from build123d import *

# Parameters (mm, degrees)
SKETCH1_R           = 5.5245
SKETCH1_R_2         = 1.7526
SKETCH1_W           = 12.7
SKETCH1_H           = 5.842
BOSS_EXTRUDE1_DEPTH = 5.842
FILLET1_R           = 1.5875
FILLET2_R           = 1.5875
FILLET3_R           = 3.175
CUT_EXTRUDE3_DEPTH  = 95.62556025


with BuildPart() as part:
    # Sketch1 → Boss-Extrude1 (new body)
    with BuildSketch(Plane(origin=(0, 0, 0), x_dir=(1, 0, 0), z_dir=(0, 1, 0))):
        with BuildLine():
            Line((-25.4, 57.15), (-12.411023526, -2.693788234))
            ThreePointArc((-12.411023526, -2.693788234), (-9.884908198, -7.97361837), (-5.259246403, -11.559858445))
            Line((-5.259246403, -11.559858445), (42.490805524, -33.284111388))
            Line((42.490805524, -33.284111388), (54.997863988, -35.489443244))
            Line((54.997863988, -35.489443244), (63.819191413, 14.538790609))
            Line((63.819191413, 14.538790609), (51.31213295, 16.744122465))
            Line((51.31213295, 16.744122465), (17.03122895, 18.5927693))
            Line((17.03122895, 18.5927693), (25.4, 57.15))
            Line((25.4, 57.15), (25.4, 69.85))
            Line((25.4, 69.85), (-25.4, 69.85))
            Line((-25.4, 69.85), (-25.4, 57.15))
        make_face()
        with Locations(Location((0, 0, 0), (0, 0, 270))):
            Circle(SKETCH1_R, mode=Mode.SUBTRACT)
        with Locations(Location((0, 63.5, 0), (0, 0, 270))):
            Circle(SKETCH1_R_2, mode=Mode.SUBTRACT)
        with Locations(Location((53.154998469, -9.37266039, 0), (0, 0, 270))):
            Circle(SKETCH1_R_2, mode=Mode.SUBTRACT)
        with Locations((-12.7, 63.5)):
            Rectangle(SKETCH1_W, SKETCH1_H, mode=Mode.SUBTRACT)
        with Locations((12.7, 63.5)):
            Rectangle(SKETCH1_W, SKETCH1_H, mode=Mode.SUBTRACT)
        Polygon((53.603383206, 9.991624401), (51.364030551, -2.708375599), (57.117277444, -3.722828253), (59.356630099, 8.977171747), align=None, mode=Mode.SUBTRACT)
        Polygon((52.706613732, -28.73694518), (54.945966387, -16.03694518), (49.192719493, -15.022492526), (46.953366838, -27.722492526), align=None, mode=Mode.SUBTRACT)
        with BuildLine():
            Line((-4.04068235, 18.616535288), (-11.026040035, 50.8))
            Line((-11.026040035, 50.8), (11.026040035, 50.8))
            Line((11.026040035, 50.8), (4.04068235, 18.616535288))
            ThreePointArc((4.04068235, 18.616535288), (0, 19.05), (-4.04068235, 18.616535288))
        make_face(mode=Mode.SUBTRACT)
        with BuildLine():
            Line((17.339787668, -7.888869605), (38.799209797, -17.651998555))
            Line((38.799209797, -17.651998555), (42.496670214, 3.317341488))
            Line((42.496670214, 3.317341488), (18.99222283, 1.48255589))
            ThreePointArc((18.99222283, 1.48255589), (18.760587695, -3.307997785), (17.339787668, -7.888869605))
        make_face(mode=Mode.SUBTRACT)
    extrude(amount=BOSS_EXTRUDE1_DEPTH)

    # Fillet1
    fillet1_edges = [part.edges().sort_by_distance(p)[0] for p in [
        (18.99222283, 2.921, -1.48255589),
        (17.339787668, 2.921, 7.888869605),
        (38.799209797, 2.921, 17.651998555),
        (42.496670214, 2.921, -3.317341488),
        (-4.04068235, 2.921, -18.616535288),
        (4.04068235, 2.921, -18.616535288),
        (11.026040035, 2.921, -50.8),
        (-11.026040035, 2.921, -50.8),
    ]]
    fillet(fillet1_edges, radius=FILLET1_R)

    # Fillet2
    fillet2_edges = [part.edges().sort_by_distance(p)[0] for p in [
        (-25.4, 2.921, -69.85),
        (25.4, 2.921, -69.85),
        (63.819191413, 2.921, -14.538790609),
        (54.997863988, 2.921, 35.489443244),
    ]]
    fillet(fillet2_edges, radius=FILLET2_R)

    # Fillet3
    fillet3_edges = [part.edges().sort_by_distance(p)[0] for p in [
        (25.4, 2.921, -57.15),
        (17.03122895, 2.921, -18.5927693),
        (51.31213295, 2.921, -16.744122465),
        (42.490805524, 2.921, 33.284111388),
        (-25.4, 2.921, -57.15),
    ]]
    fillet(fillet3_edges, radius=FILLET3_R)

    # Sketch2 → Cut-Extrude3 (cut, through all)
    with BuildSketch(Plane(origin=(0, 5.842, 0), x_dir=(1, 0, 0), z_dir=(0, 1, 0))):
        with BuildLine():
            Line((1.5875, 54.791775853), (-1.5875, 54.791775853))
            ThreePointArc((-1.5875, 54.791775853), (-3.96875, 57.173025853), (-1.5875, 59.554275853))
            Line((-1.5875, 59.554275853), (1.5875, 59.554275853))
            ThreePointArc((1.5875, 59.554275853), (3.96875, 57.173025853), (1.5875, 54.791775853))
        make_face()
    extrude(amount=-CUT_EXTRUDE3_DEPTH, mode=Mode.SUBTRACT)


solid = part.part
Input: part model. Units: mm. Frame: model coordinates. A direction names the side the tool comes from. Give positions to 0.01 mm unless a question says otherwise; leave off trailing zeros. Write each loop counter-clockwise with the first axis right and the second up, starting at its lowest first coordinate (ties: lowest second). Pieces come first, ordered by that corner, then holes. Notation, with made-up numbers: M 51,36.25 L 68,36.25 A16 ccw 68,45.25 Z; hole C 1.5,-25.75 d4. An arc over 180 degrees is marked long. Write item = value, one per line. Start each with the question number.
1) Cut plane A-A on x = 0. Return the cut outline in (y, z).
2) Draft query along Z for faces 1 (the flat face through (59.35, 2.88, 10.8)), 2 (the flat face through (30.62, 2.88, -2.39)), 3 (the flat face through (18, 0, -18)). Return one class per face: +Z half, -Z half, draft (parallel to the pull), parting line (faces both ways), or undercut.
3) First-contact query: pin 1 Ø1.8 at (x, y) = (12.5, 2) entering from +Z; pin 2 Ø2 at (y, z) = (4, 21) entering from +X; pin 3 Ø3.5 at (x, y) = (-0.5, 4) entering from +Z. Flat tips, straight axial feed; report the tip coordinate or a pass-through.
4) Material intervals for line 1 along X through (y, z) = (4.5, -66); line 2 along X through (y, z) = (3.35, -62.5); line 3 along X through (y, z) = (4.65, 9), sorted ascending. Write a range as [from, to].
5) Cut plane D-D on z = 21.5. Return the cut outline in (x, y).
6) Cut plane C-C on x = 34. Return the cut outline in (y, z).
7) Cut plane B-B on z = -63.5. Return the cut outline in (x, y), then the cut area to 3 significant figures.
8) Reachability of faces 4 (the flat face through (25.4, 3, -63)), 5 (the flat face through (21.52, 2.88, -39.28)), 6 (the flat face through (-25.4, 3, -63)), 7 (the flat face through (7.53, 2.88, -34.69)) from +Z, -Z, +X, -X, +Y, -Y: full face, straight path, thin tool, end or side. Return the list, or none.
Solved:
q1.outline = M 0,-69.85 L 5.84,-69.85 L 5.84,-65.25 L 0,-65.25 Z; M 0,-61.75 L 5.84,-61.75 L 5.84,-59.55 L 0,-59.55 Z; M 0,-54.79 L 5.84,-54.79 L 5.84,-50.8 L 0,-50.8 Z; M 0,-19.05 L 5.84,-19.05 L 5.84,-5.52 L 0,-5.52 Z; M 0,5.52 L 5.84,5.52 L 5.84,13.95 L 0,13.95 Z
q2.face_1 = +Z half
q2.face_2 = undercut
q2.face_3 = draft
q3.pin_1 = 20.05
q3.pin_2 = 57.73
q3.pin_3 = 14.52
q4.line_1 = [-25.4, -19.05], [-6.35, 6.35], [19.05, 25.4]
q4.line_2 = [-25.4, -19.05], [-6.35, -1.44], [1.44, 6.35], [19.05, 25.4]
q4.line_3 = [-8.96, 19.78], [40.32, 51.44], [54.87, 59.67]
q5.outline = M 16.59,0 L 48.05,0 L 48.05,5.84 L 16.59,5.84 Z; M 53.98,0 L 57.46,0 L 57.46,5.84 L 53.98,5.84 Z
q6.outline = M 0,-17.68 L 5.84,-17.68 L 5.84,-2.65 L 0,-2.65 Z; M 0,15.47 L 5.84,15.47 L 5.84,29.42 L 0,29.42 Z
q7.outline = M -25.4,0 L -19.05,0 L -19.05,5.84 L -25.4,5.84 Z; M -6.35,0 L -1.75,0 L -1.75,5.84 L -6.35,5.84 Z; M 1.75,0 L 6.35,0 L 6.35,5.84 L 1.75,5.84 Z; M 19.05,0 L 25.4,0 L 25.4,5.84 L 19.05,5.84 Z
q7.area = 128 mm2
q8.face_4 = -Z, +X, +Y, -Y
q8.face_5 = +X, +Y, -Y
q8.face_6 = +Z, -Z, -X, +Y, -Y
q8.face_7 = +Y, -Y
